```python
from build123d import *

# Parameters (mm, degrees)
F0_W     = 9.525
F0_H     = 19.05
F1_DEPTH = 0.396875
F0_H_2   = 6.35
F0_R     = 1.367696
F0_R_2   = 1.5
F2_DEPTH = 1.190625
F3_DEPTH = 4.445


with BuildPart() as f1:
    # F0 (on Front) → F1 (new body, symmetric)
    with BuildSketch(Plane.XZ):
        with Locations((-25.237318, 31.262366)):
            Rectangle(F0_W, F0_H)
    extrude(amount=F1_DEPTH, both=True)

    # F0 (on Front) → F2 (join, symmetric)
    with BuildSketch(Plane.XZ):
        with Locations((-25.237318, 43.962366)):
            Rectangle(F0_W, F0_H_2)
        with Locations((-25.237318, 43.962366)):
            Circle(F0_R, mode=Mode.SUBTRACT)
        with Locations((-25.237318, 18.562366)):
            Rectangle(F0_W, F0_H_2)
        with Locations((-25.237318, 18.562366)):
            Circle(F0_R_2, mode=Mode.SUBTRACT)
    extrude(amount=F2_DEPTH, both=True)

    # F0 (on Front) → F3 (join, symmetric)
    with BuildSketch(Plane.XZ):
        with Locations((-25.237318, 43.962366)):
            Circle(F0_R)
        with Locations((-25.237318, 18.562366)):
            Circle(F0_R_2)
    extrude(amount=F3_DEPTH, both=True)


solid = f1.part
```
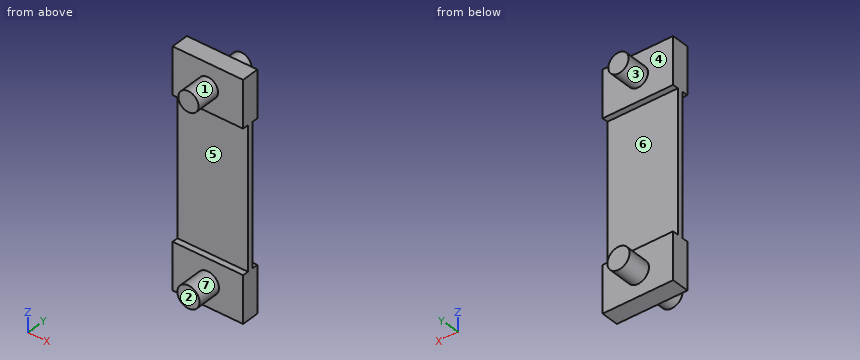
Check sheet for the modelled part. Datum: model origin and axes. Units: mm. Face numbers are marked on the shaded views. A direction names the side the tool comes from. Coordinates: 2 decimals unless noted, no trailing zeros. Order: outer loops, then holes, each group sorted by start corner. A loop starts at its lowest first (then second) coordinate and runs counter-clockwise, first axis right, second up. Notation, with made-up numbers: M 27.25,7 L 72.25,7 A10 cw 72.25,21 Z; hole C 76,28 d6. An arc over 180 degrees is marked long. One line per question, with ' | ' between items. Start each with the question number.
Item 1: Sectioned sample at D-D on x = -26. Record the cut outline in (y, z) (3 decimals).
Item 2: Access from +Z, -Z, +X, -X, +Y, -Y to the whole of each face (thin tool, end or side, straight path). Record for the marked faces 4, 5, 6 and 7.
Item 3: Gauge pin test, flat ends, axial feed: P1, Ø3, axis at x = -24, y = 3.5, coming from the -Z side; P2, Ø1, axis at y = 2, z = 44, coming from the -X side (3 decimals). Record the tip position at first contact, or that the pin passes through.
Item 4: Material ranges on line 1 (Z direction, x = -28.5, y = -0.75); line 2 (Y direction, x = -22, z = 30.5); line 3 (Y direction, x = -22.25, z = 45), recorded low to high.
Item 5: Mould release check, pull along Z, two halves, no side actions. Record for the marked faces 1, 2 and 3: pulls with the +Z half, pulls with the -Z half, needs draft (parallel to the pull), parting line crosses it, or undercut.
Item 6: Sectioned sample at B-B on x = -22.5. Record the cut outline in (y, z).
Item 7: Sectioned sample at C-C on z = 18. Record the cut outline in (x, y) (3 decimals).
Item 8: Sectioned sample at A-A on y = 0.75. Record the cut outline in (x, z), and give its area (3 significant figures).
Answer below:
1) outline: M -4.445,17.271 L -1.191,17.271 L -1.191,15.387 L 1.191,15.387 L 1.191,17.271 L 4.445,17.271 L 4.445,19.854 L 1.191,19.854 L 1.191,21.737 L 0.397,21.737 L 0.397,40.787 L 1.191,40.787 L 1.191,42.827 L 4.445,42.827 L 4.445,45.098 L 1.191,45.098 L 1.191,47.137 L -1.191,47.137 L -1.191,45.098 L -4.445,45.098 L -4.445,42.827 L -1.191,42.827 L -1.191,40.787 L -0.397,40.787 L -0.397,21.737 L -1.191,21.737 L -1.191,19.854 L -4.445,19.854 Z
2) face 4: +Y | face 5: +X, -X, -Y | face 6: +X, -X, +Y | face 7: -Y
3) P1: stops at z = 17.06 | P2: stops at x = -26.605
4) line 1: z = 15.39 to 21.74, 40.79 to 47.14 | line 2: y = -0.4 to 0.4 | line 3: y = -1.19 to 1.19
5) face 1: undercut | face 2: needs draft | face 3: undercut
6) outline: M -1.19,15.39 L 1.19,15.39 L 1.19,21.74 L 0.4,21.74 L 0.4,40.79 L 1.19,40.79 L 1.19,47.14 L -1.19,47.14 L -1.19,40.79 L -0.4,40.79 L -0.4,21.74 L -1.19,21.74 Z
7) outline: M -30,-1.191 L -26.628,-1.191 L -26.628,-4.445 L -23.847,-4.445 L -23.847,-1.191 L -20.475,-1.191 L -20.475,1.191 L -23.847,1.191 L -23.847,4.445 L -26.628,4.445 L -26.628,1.191 L -30,1.191 Z
8) outline: M -30,15.39 L -20.47,15.39 L -20.47,21.74 L -30,21.74 Z; M -30,40.79 L -20.47,40.79 L -20.47,47.14 L -30,47.14 Z | area: 121 mm^2
